from build123d import *

# Parameters (mm, degrees)
SKETCH_R            = 2.5
PAD_DEPTH           = 2
SKETCH001_W         = 50
SKETCH001_H         = 10
SKETCH001_W_2       = 55
POCKET_DEPTH        = 5
LINEARPATTERN_COUNT = 10
LINEARPATTERN_PITCH = 15.555556


with BuildPart() as part:
    # Sketch → Pad (new body)
    with BuildSketch(Plane.XY):
        Polygon((-47.5, 227.5), (47.5, 227.5), (107.5, 167.5), (107.5, -167.5), (47.5, -227.5), (-47.5, -227.5), (-107.5, -167.5), (-107.5, 167.5), align=None)
        with Locations((-97.5, 157.5)):
            Circle(SKETCH_R, mode=Mode.SUBTRACT)
        with Locations((-37.5, 217.5)):
            Circle(SKETCH_R, mode=Mode.SUBTRACT)
        with Locations((37.5, 217.5)):
            Circle(SKETCH_R, mode=Mode.SUBTRACT)
        with Locations((97.5, 157.5)):
            Circle(SKETCH_R, mode=Mode.SUBTRACT)
        with Locations((97.5, -157.5)):
            Circle(SKETCH_R, mode=Mode.SUBTRACT)
        with Locations((37.5, -217.5)):
            Circle(SKETCH_R, mode=Mode.SUBTRACT)
        with Locations((-37.5, -217.5)):
            Circle(SKETCH_R, mode=Mode.SUBTRACT)
        with Locations((-97.5, -157.5)):
            Circle(SKETCH_R, mode=Mode.SUBTRACT)
    extrude(amount=PAD_DEPTH)

    # Sketch001 → Pocket (cut)
    with BuildSketch(Plane.XY.offset(2)):
        with Locations((-62.5, 142.5)):
            Rectangle(SKETCH001_W, SKETCH001_H)
        with Locations((62.5, 142.5)):
            Rectangle(SKETCH001_W, SKETCH001_H)
        with Locations((0, 142.5)):
            Rectangle(SKETCH001_W_2, SKETCH001_H)
    pocket = extrude(amount=-POCKET_DEPTH, mode=Mode.SUBTRACT)

    # LinearPattern: Pocket ×10
    with Locations(*[(0, -i * LINEARPATTERN_PITCH, 0) for i in range(1, LINEARPATTERN_COUNT)]):
        add(pocket, mode=Mode.SUBTRACT)


solid = part.part
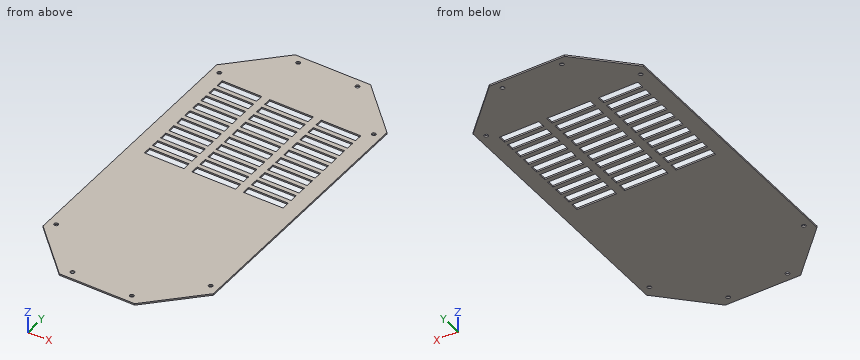
Geometry check sheet. Reference: the model listing, model coordinates, mm. Coordinates: 2 decimals unless noted, no trailing zeros. One line per question, with ' | ' between items.
1. Depth check by flat-ended pin: pin 1 Ø0.6 at (x, z) = (-53.5, 0.5) entering from -Y. Enter the tip coordinate at first touch or a pass-through.
Answers:
pin 1: stops at y = -221.8
2. Cross-section at A-A on x = -18. State how many separate pieces and enclosed holes the cut face has, and give its area (3 significant figures).
Answers:
separate pieces: 11 | enclosed holes: 0 | area: 710 mm²
3. Thickness scan on probe 1 along X at (y, z) = (157.5, 0.45); probe 2 along X at (y, z) = (44.5, 0.75); probe 3 along X at (y, z) = (-217.5, 0.6). Record the ranges inside material, lowest first. Write a range as from..to.
Answers:
probe 1: x = -107.5..-100, -95..95, 100..107.5 | probe 2: x = -107.5..-87.5, -37.5..-27.5, 27.5..37.5, 87.5..107.5 | probe 3: x = -57.5..-40, -35..35, 40..57.5
